Verification items for this drawing (mm, ordinates from the low corner). Coordinates: 2 decimals unless noted, no trailing zeros. Order: outer loops, then holes, each group sorted by start corner. A loop starts at its lowest first (then second) coordinate and runs counter-clockwise, first axis right, second up. Notation, with made-up numbers: (88, -4) -> (131, -4) arc R28 ccw to (131, 27) -> close; hole circle Ø10 at (-3, 58). An arc over 180 degrees is marked (long way). Answer in a Markdown table with one row per item. Add a question column.
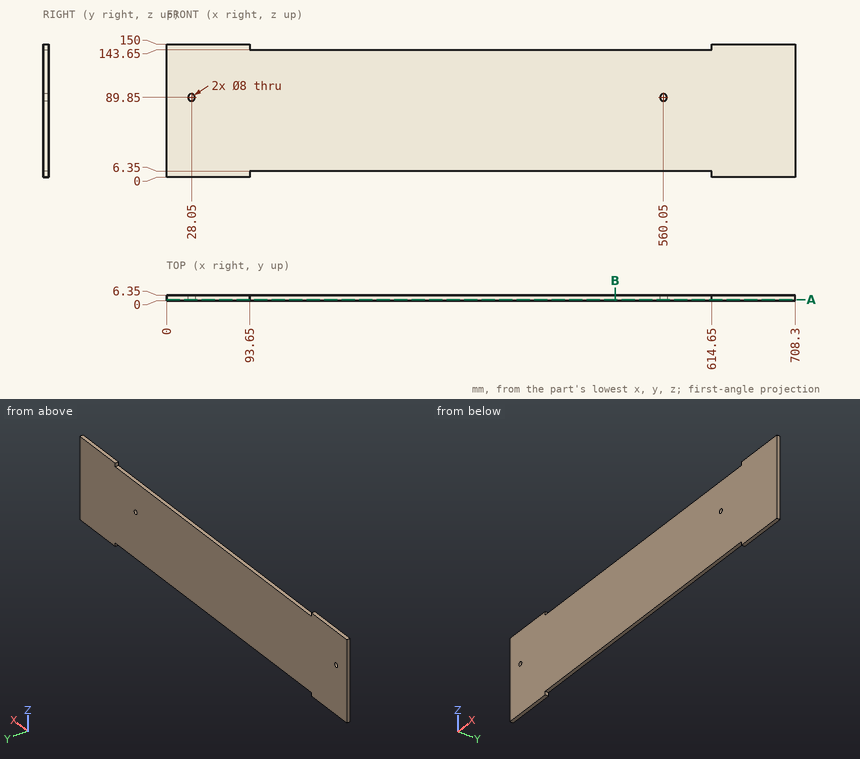
(1) Cross-section at A-A (y = 1.25). Enter the section's corners in (x, z), plus the area to 3 significant figures.
(2) Scan lines: line 1 along X through (y, z) = (3.25, 89.85); line 2 along Z through (x, y) = (560.05, 3.5); line 3 along Z through (x, y) = (28.05, 2.5). Record each from-to range of solid material in increasing order.
(3) Go/stop test with flat-tipped pins: P1, Ø6.5, axis at x = 560.05, z = 89.85, coming from the -Y side; P2, Ø2, axis at x = 484, y = 1.5, coming from the -Z side; P3, Ø3, axis at x = 349, y = 0.5, coming from the +Z side. Record where each tip stops, or that it passes through.
(4) Cross-section at B-B (x = 505.5). Enter the section's corners in (y, z), plus the area to 3 significant figures.
Checks:
| question | item | result |
|---|---|---|
| 1 | outline | (0, 0) -> (93.65, 0) -> (93.65, 6.35) -> (614.65, 6.35) -> (614.65, 0) -> (708.3, 0) -> (708.3, 150) -> (614.65, 150) -> (614.65, 143.65) -> (93.65, 143.65) -> (93.65, 150) -> (0, 150) -> close; hole circle Ø8 at (28.05, 89.85); hole circle Ø8 at (560.05, 89.85) |
| 1 | area | 99,500 mm² |
| 2 | line 1 | 0 to 24.05, 32.05 to 556.05, 564.05 to 708.3 |
| 2 | line 2 | 6.35 to 85.85, 93.85 to 143.65 |
| 2 | line 3 | 0 to 85.85, 93.85 to 150 |
| 3 | P1 | through |
| 3 | P2 | z = 6.35 |
| 3 | P3 | z = 143.65 |
| 4 | outline | (0, 6.35) -> (6.35, 6.35) -> (6.35, 143.65) -> (0, 143.65) -> close |
| 4 | area | 872 mm² |
